The model under review builds one solid part; all positions refer to its coordinate system, in mm. A direction names the side the tool comes from. Round coordinates to 2 decimals unless told otherwise and drop trailing zeros. Loops run counter-clockwise (first coordinate to the right, second up) from the corner with the lowest first, then second, coordinate; pieces in that order, holes last. Notation, with made-up numbers: M 27,-33 L 57,-33 A21 ccw 57,-26 Z; hole C 51,-7.75 d9. An arc over 180 degrees is marked long. Return JSON: item names as keys, results as strings. Group by question number.
Q1. To check wall thickness, follow line 1 along X through (y, z) = (6.5, 61); line 2 along X through (y, z) = (2.5, 25); line 3 along X through (y, z) = (3.5, 12.5). State the ranges of each line that lie inside material, in increasing order.
Q2. Consider section A-A (y = 4). Count the separate pieces of the cut face and the enclosed holes in it, and give its area (3 significant figures).
Q3. Consider section D-D (x = 25). State the section outline as (y, z) points, and give its area (3 significant figures).
Q4. Clearance check with flat-ended pins moving along their axes: pin 1 Ø1.5 at (x, z) = (51.76, 15.24) entering from -Y; pin 2 Ø3 at (x, y) = (8, 5) entering from -Z; pin 3 Ø3.5 at (x, y) = (56, 5) entering from +Z; pin 4 Ø7.5 at (x, z) = (66, 48.5) entering from +Y. State where each tip first meets the part, or that it passes through.
Q5. Consider section B-B (z = 6). State the section outline as (x, y) points.
Q6. Consider section C-C (x = 45). State the section outline as (y, z) points.
Q7. Draft analysis for pull direction X (two halves, no side actions). For faces 5 (the face through (59.391, 5, 39)), 6 (the face through (64.1, 1.5, 3)), 7 (the face through (34, 0, 40)), state which applies: pulls with the +X half, pulls with the -X half, needs draft (parallel to the pull), parting line crosses it, or undercut.
Q8. For faces 1 (the face through (3, 5, 38)), 2 (the face through (54, 3, 77.366)), 3 (the face through (4.416, 4.972, 76.023)), 4 (the face through (62.391, 1, 39)), list the 3-axis set-ups (+Z, -Z, +X, -X, +Y, -Y) from which the entire face can be reached by the end or side of a thin tool; tool diameter is ignored.
from build123d import *

# Parameters (mm, degrees)
CROQUIS2_R              = 0.95
SALIENTE_EXTRUIR1_DEPTH = 3
SALIENTE_EXTRUIR2_DEPTH = 4
CROQUIS5_R              = 1.95
CROQUIS5_R_2            = 0.95
SALIENTE_EXTRUIR3_DEPTH = 2.5


with BuildPart() as part:
    # Croquis2 → Saliente-Extruir1 (new body)
    # profile 1 of 9: a face of its own
    with BuildSketch(Plane(origin=(0, 0, 0), x_dir=(1, 0, 0), z_dir=(0, 1, 0))):
        Polygon((42.257715083, -74.365742034), (56.391047804, -74.365742034), (56.391047804, 0), (3, 0), (3, -74.607271369), (5.792893219, -77.400164587), (39.10235492, -77.400164587), align=None)
        with Locations((5.766718429, -14.088511522)):
            Circle(CROQUIS2_R, mode=Mode.SUBTRACT)
        with Locations((51.762416691, -15.240864439)):
            Circle(CROQUIS2_R, mode=Mode.SUBTRACT)
        with Locations((10.912444351, -74.653169117)):
            Circle(CROQUIS2_R, mode=Mode.SUBTRACT)
        with Locations((37.82696283, -74.653169117)):
            Circle(CROQUIS2_R, mode=Mode.SUBTRACT)
    # profile 2 of 9: a face of its own
    with BuildSketch(Plane(origin=(0, 0, 0), x_dir=(1, 0, 0), z_dir=(0, 1, 0))):
        Polygon((3, 0), (0, 0), (0, -75.849912056), (4.550252532, -80.400164587), (40.310801486, -80.400164587), (43.466161649, -77.365742034), (59.391047804, -77.365742034), (59.391047804, -72.615742034), (59.391047804, -4.75), (59.391047804, 0), (56.391047804, 0), (56.391047804, -74.365742034), (42.257715083, -74.365742034), (39.10235492, -77.400164587), (5.792893219, -77.400164587), (3, -74.607271369), align=None)
    # profile 3 of 9: a face of its own
    with BuildSketch(Plane(origin=(0, 0, 0), x_dir=(1, 0, 0), z_dir=(0, 1, 0))):
        with Locations((5.766718429, -14.088511522)):
            Circle(CROQUIS2_R)
    # profile 4 of 9: a face of its own
    with BuildSketch(Plane(origin=(0, 0, 0), x_dir=(1, 0, 0), z_dir=(0, 1, 0))):
        with Locations((37.82696283, -74.653169117)):
            Circle(CROQUIS2_R)
    # profile 5 of 9: a face of its own
    with BuildSketch(Plane(origin=(0, 0, 0), x_dir=(1, 0, 0), z_dir=(0, 1, 0))):
        with BuildLine():
            ThreePointArc((64.141047804, 0), (60.782290593, -1.391242789), (59.391047804, -4.75))
            Line((59.391047804, -4.75), (59.391047804, -72.615742034))
            ThreePointArc((59.391047804, -72.615742034), (60.782290593, -75.974499245), (64.141047804, -77.365742034))
            ThreePointArc((64.141047804, -77.365742034), (67.499805014, -75.974499245), (68.891047804, -72.615742034))
            Line((68.891047804, -72.615742034), (68.891047804, -4.75))
            ThreePointArc((68.891047804, -4.75), (67.499805014, -1.391242789), (64.141047804, 0))
        make_face()
        with BuildLine():
            ThreePointArc((62.391047804, -4.75), (64.141047804, -3), (65.891047804, -4.75))
            Line((65.891047804, -4.75), (65.891047804, -72.615742034))
            ThreePointArc((65.891047804, -72.615742034), (64.141047804, -74.365742034), (62.391047804, -72.615742034))
            Line((62.391047804, -72.615742034), (62.391047804, -4.75))
        make_face(mode=Mode.SUBTRACT)
    # profile 6 of 9: a face of its own
    with BuildSketch(Plane(origin=(0, 0, 0), x_dir=(1, 0, 0), z_dir=(0, 1, 0))):
        with Locations((51.762416691, -15.240864439)):
            Circle(CROQUIS2_R)
    # profile 7 of 9: a face of its own
    with BuildSketch(Plane(origin=(0, 0, 0), x_dir=(1, 0, 0), z_dir=(0, 1, 0))):
        with Locations((10.912444351, -74.653169117)):
            Circle(CROQUIS2_R)
    # profile 8 of 9: a face of its own
    with BuildSketch(Plane(origin=(0, 0, 0), x_dir=(1, 0, 0), z_dir=(0, 1, 0))):
        with BuildLine():
            Line((59.391047804, -72.615742034), (59.391047804, -77.365742034))
            Line((59.391047804, -77.365742034), (64.141047804, -77.365742034))
            ThreePointArc((64.141047804, -77.365742034), (60.782290593, -75.974499245), (59.391047804, -72.615742034))
        make_face()
    # profile 9 of 9: a face of its own
    with BuildSketch(Plane(origin=(0, 0, 0), x_dir=(1, 0, 0), z_dir=(0, 1, 0))):
        with BuildLine():
            Line((64.141047804, 0), (59.391047804, 0))
            Line((59.391047804, 0), (59.391047804, -4.75))
            ThreePointArc((59.391047804, -4.75), (60.782290593, -1.391242789), (64.141047804, 0))
        make_face()
    extrude(amount=SALIENTE_EXTRUIR1_DEPTH)

    # Croquis4 → Saliente-Extruir2 (add)
    with BuildSketch(Plane(origin=(0, 3, 0), x_dir=(1, 0, 0), z_dir=(0, 1, 0))):
        Polygon((0, 0), (0, -75.849912056), (4.550252532, -80.400164587), (40.310801486, -80.400164587), (43.466161649, -77.365742034), (59.391047804, -77.365742034), (59.391047804, 0), (56.391047804, 0), (56.391047804, -74.365742034), (42.257715083, -74.365742034), (39.10235492, -77.400164587), (5.792893219, -77.400164587), (3, -74.607271369), (3, 0), align=None)
    extrude(amount=SALIENTE_EXTRUIR2_DEPTH)

    # Croquis5 → Saliente-Extruir3 (add)
    # profile 1 of 4: a face of its own
    with BuildSketch(Plane(origin=(0, 3, 0), x_dir=(1, 0, 0), z_dir=(0, 1, 0))):
        with Locations(Location((5.766718429, -14.088511522, 0), (0, 0, 270))):
            Circle(CROQUIS5_R)
        with Locations(Location((5.766718429, -14.088511522, 0), (0, 0, 270))):
            Circle(CROQUIS5_R_2, mode=Mode.SUBTRACT)
    # profile 2 of 4: a face of its own
    with BuildSketch(Plane(origin=(0, 3, 0), x_dir=(1, 0, 0), z_dir=(0, 1, 0))):
        with Locations(Location((51.762416691, -15.240864439, 0), (0, 0, 270))):
            Circle(CROQUIS5_R)
        with Locations(Location((51.762416691, -15.240864439, 0), (0, 0, 270))):
            Circle(CROQUIS5_R_2, mode=Mode.SUBTRACT)
    # profile 3 of 4: a face of its own
    with BuildSketch(Plane(origin=(0, 3, 0), x_dir=(1, 0, 0), z_dir=(0, 1, 0))):
        with Locations(Location((37.82696283, -74.653169117, 0), (0, 0, 270))):
            Circle(CROQUIS5_R)
        with Locations(Location((37.82696283, -74.653169117, 0), (0, 0, 270))):
            Circle(CROQUIS5_R_2, mode=Mode.SUBTRACT)
    # profile 4 of 4: a face of its own
    with BuildSketch(Plane(origin=(0, 3, 0), x_dir=(1, 0, 0), z_dir=(0, 1, 0))):
        with Locations(Location((10.912444351, -74.653169117, 0), (0, 0, 270))):
            Circle(CROQUIS5_R)
        with Locations(Location((10.912444351, -74.653169117, 0), (0, 0, 270))):
            Circle(CROQUIS5_R_2, mode=Mode.SUBTRACT)
    extrude(amount=SALIENTE_EXTRUIR3_DEPTH)


solid = part.part
Values:
{
 "1": {"line 1": "x = 0 to 3, 56.39 to 59.39", "line 2": "x = 0 to 62.39, 65.89 to 68.89", "line 3": "x = 0 to 3, 4.64 to 6.9, 56.39 to 59.39"},
 "2": {"separate pieces": "5", "enclosed holes": "4", "area": "667 mm2"},
 "3": {"outline": "M 0,0 L 3,0 L 3,77.4 L 7,77.4 L 7,80.4 L 0,80.4 Z", "area": "253 mm2"},
 "4": {"pin 1": "stops at y = 0", "pin 2": "stops at z = 12.28", "pin 3": "stops at z = 77.37", "pin 4": "stops at y = 3"},
 "5": {"outline": "M 0,0 L 62.39,0 L 62.39,3 L 59.39,3 L 59.39,7 L 56.39,7 L 56.39,3 L 3,3 L 3,7 L 0,7 Z; M 65.89,0 L 68.89,0 L 68.89,3 L 65.89,3 Z"},
 "6": {"outline": "M 0,0 L 3,0 L 3,74.37 L 7,74.37 L 7,77.37 L 0,77.37 Z"},
 "7": {"face 5": "pulls with the +X half", "face 6": "undercut", "face 7": "needs draft"},
 "8": {"face 1": "-Z, +Y", "face 2": "+Z, +X, +Y, -Y", "face 3": "+Y", "face 4": "+Y, -Y"}
}
